The drawing under review shows one solid part. Ordinate dimensions are in mm from its lowest x, y, z. A direction names the side the tool comes from. Round coordinates to 2 decimals unless told otherwise and drop trailing zeros. Order: outer loops, then holes, each group sorted by start corner. A loop starts at its lowest first (then second) coordinate and runs counter-clockwise, first axis right, second up. Notation, with made-up numbers: M 14,88.5 L 48,88.5 A14 ccw 48,107.5 Z; hole C 8,58.25 d4. An arc over 180 degrees is marked long. Answer as a JSON object with one key per item and string values.
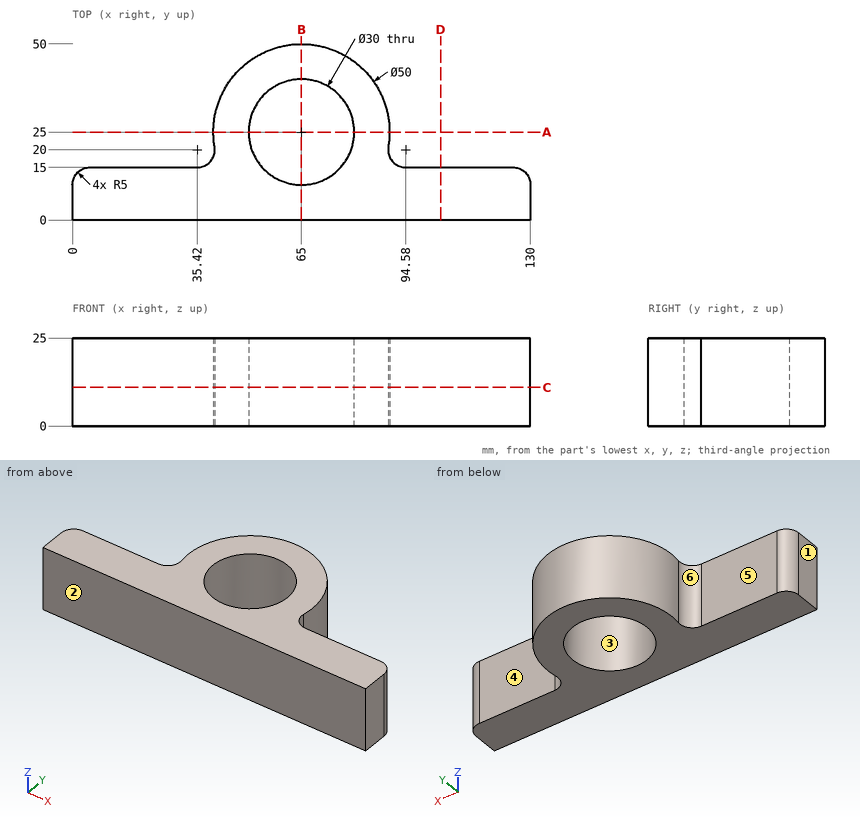
1) Add section D-D on x = 104.5. State the section outline as (y, z) points.
Geometry check:
{"outline": "M 0,0 L 15,0 L 15,25 L 0,25 Z"}
2) Insertion check: P1, Ø1.5, axis at y = 13, z = 8.5, coming from the -X side (1 decimal); P2, Ø12, axis at x = 57, y = 18, coming from the -Z side; P3, Ø12.5, axis at x = 18.5, z = 10.5, coming from the +Y side; P4, Ø6, axis at y = 23, z = 15, coming from the -X side. Each pin has a flat end and moves straight along its axis. Give the tip position at first contact, or say it passes through.
Geometry check:
{"P1": "stops at x = 0.5", "P2": "stops at z = 0", "P3": "stops at y = 15", "P4": "stops at x = 40"}
3) Add section A-A on y = 25. State the section outline as (x, z) points.
Geometry check:
{"outline": "M 40,0 L 50,0 L 50,25 L 40,25 Z; M 80,0 L 90,0 L 90,25 L 80,25 Z"}
4) Machinability: for the marked faces 4, 5 and 6, which of the approach directions +Z, -Z, +X, -X, +Y, -Y give a long, thin tool a straight path to every point of the face, cutting with its end or side? Answer none if there is none.
Geometry check:
{"face 4": "+Z, -Z, +X, +Y", "face 5": "+Z, -Z, -X, +Y", "face 6": "+Z, -Z, -X"}
5) Mouldability with a two-part tool opening along Y and no side actions: class the marked faces 1, 2 and 3 as +Y half, -Y half, draft (parallel to the pull), parting line (faces both ways), or undercut.
Geometry check:
{"face 1": "draft", "face 2": "-Y half", "face 3": "undercut"}
6) Add section B-B on x = 65. State the section outline as (y, z) points.
Geometry check:
{"outline": "M 0,0 L 10,0 L 10,25 L 0,25 Z; M 40,0 L 50,0 L 50,25 L 40,25 Z"}
7) For L1, parallel to Y at x = 101.5, z = 22; L2, parallel to Y at x = 56, z = 18.25 (1 decimal); L3, parallel to X at y = 20, z = 19, list the stretches that pass through material, from the lowest coordinate up.
Geometry check:
{"L1": "y = 0 to 15", "L2": "y = 0 to 13, 37 to 48.3", "L3": "x = 40.42 to 50.86, 79.14 to 89.58"}
8) Add section C-C on z = 11. State the section outline as (x, y) points, and give its area (3 significant figures).
Geometry check:
{"outline": "M 0,0 L 130,0 L 130,10 A5 ccw 125,15 L 94.58,15 A5 cw 89.65,20.83 A25 ccw long 40.35,20.83 A5 cw 35.42,15 L 5,15 A5 ccw 0,10 Z; hole C 65,25 d30", "area": "2,720 mm²"}
